```python
from build123d import *

# Parameters (mm, degrees)
SKETCH1_R           = 2
BOSS_EXTRUDE1_DEPTH = 100
BOSS_EXTRUDE2_DEPTH = 3
FILLET2_R           = 0.2


with BuildPart() as part:
    # Sketch1 → Boss-Extrude1 (new body)
    with BuildSketch(Plane(origin=(0, 0, 0), x_dir=(1, 0, 0), z_dir=(0, 1, 0))):
        with Locations(Location((0, 0, 0), (0, 0, 270))):
            Circle(SKETCH1_R)
    extrude(amount=BOSS_EXTRUDE1_DEPTH)

    # Sketch2 → Boss-Extrude2 (add)
    with BuildSketch(Plane.XZ):
        Polygon((3.983716857, 0), (1.991858429, 3.45), (-1.991858429, 3.45), (-3.983716857, 0), (-1.991858429, -3.45), (1.991858429, -3.45), align=None)
    extrude(amount=BOSS_EXTRUDE2_DEPTH)

    # Fillet2
    fillet2_edges = [part.edges().sort_by_distance(p)[0] for p in [
        (0, 0, -2),
        (2.987787643, 0, -1.725),
        (2.987787643, 0, 1.725),
        (0, 0, 3.45),
        (-2.987787643, 0, 1.725),
        (-2.987787643, 0, -1.725),
        (0, 0, -3.45),
        (2.987787643, -3, -1.725),
        (2.987787643, -3, 1.725),
        (0, -3, 3.45),
        (-2.987787643, -3, 1.725),
        (-2.987787643, -3, -1.725),
        (0, -3, -3.45),
    ]]
    fillet(fillet2_edges, radius=FILLET2_R)


solid = part.part
```
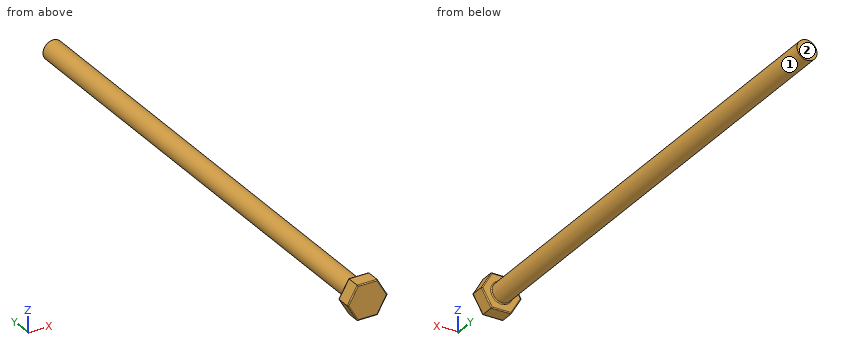
CAD build for the part. Positions are in the model's coordinates, mm. Face numbers are marked on the shaded views. A direction names the side the tool comes from. Coordinates: 2 decimals unless noted, no trailing zeros. Loops run counter-clockwise (first coordinate to the right, second up) from the corner with the lowest first, then second, coordinate; pieces in that order, holes last. Notation, with made-up numbers: (-24.75, 41) - (20.25, 41) arc R20 ccw to (20.25, 69) - close; hole circle Ø4 at (57.25, 31.25). An arc over 180 degrees is marked (long way). Use CSV: the item, a comma, the result in double quotes. Start each with the question number.
Q1. Cut at A-A, the plane x = 0. List the corners of the cut face in (y, z), then the cut area to 3 significant figures.
Q2. Probe probe 1 along X at (y, z) = (81.5, 0); probe 2 along X at (y, z) = (57, 1.75); probe 3 along Y at (x, z) = (0.5, -2.75). List the from-to ranges inside material, lowest first. Write a range as from..to.
Q3. 3-axis set-ups, long thin cutter, end or side, ignore diameter. For the marked faces 1 and 2: which of +Z, -Z, +X, -X, +Y, -Y reach the whole face in a straight line?
Q4. Cut at B-B, the plane y = 78. List the corners of the cut face in (x, z), then the cut area to 3 significant figures.
Q5. Drop flat-ended pins along their axis: P1, Ø4, axis at y = 48, z = 2.5, coming from the -X side; P2, Ø4, axis at x = 1, y = 69, coming from the -Z side; P3, Ø1.5, axis at y = 31.5, z = 0.5, coming from the -X side. Give the stop position or say it passes through.
Here are the results:
1,outline,"(-3, -3.25) arc R0.2 ccw to (-2.8, -3.45) - (-0.2, -3.45) arc R0.2 ccw to (0, -3.25) - (0, -2.2) arc R0.2 cw to (0.2, -2) - (100, -2) - (100, 2) - (0.2, 2) arc R0.2 cw to (0, 2.2) - (0, 3.25) arc R0.2 ccw to (-0.2, 3.45) - (-2.8, 3.45) arc R0.2 ccw to (-3, 3.25) - close"
1,area,"421 mm2"
2,probe 1,"-2..2"
2,probe 2,"-0.97..0.97"
2,probe 3,"-3..0"
3,face 1,"+Y"
3,face 2,"+Z, -Z, +X, -X, +Y"
4,outline,"circle Ø4 at (0, 0)"
4,area,"12.6 mm2"
5,P1,"x = -1.94"
5,P2,"z = -2"
5,P3,"x = -2"
